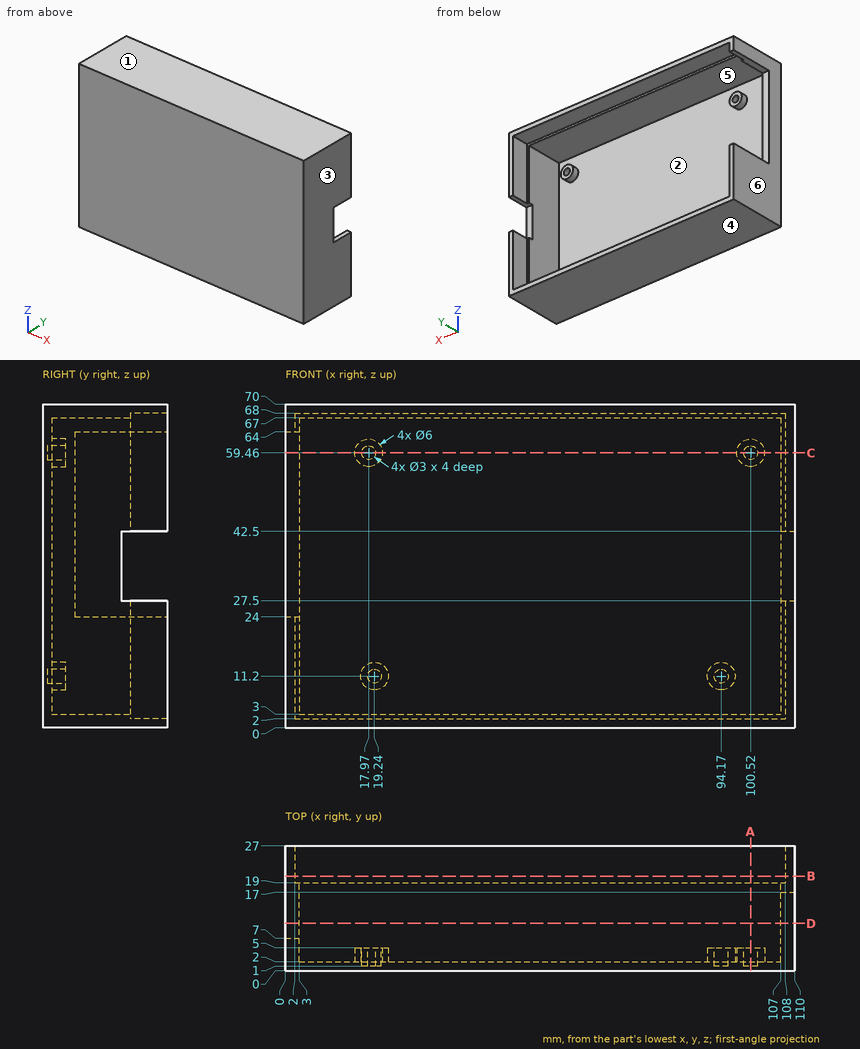
For this review, use the dimensioned drawing (mm, ordinates from the lowest corner) and the shaded views. A direction names the side the tool comes from. Coordinates: 2 decimals unless noted, no trailing zeros. Order: outer loops, then holes, each group sorted by start corner. A loop starts at its lowest first (then second) coordinate and runs counter-clockwise, first axis right, second up. Notation, with made-up numbers: (-9.75, 55.25) - (18.25, 55.25) arc R23 ccw to (18.25, 90.25) - close; hole circle Ø2 at (40.5, -28). An arc over 180 degrees is marked (long way). Use one line per item in the form item = value.
Q1. For probe 1 along X at (y, z) = (2.05, 11.2); probe 2 along X at (y, z) = (2.55, 59.46); probe 3 along X at (y, z) = (1.9, 11.2), list the stretches that pass through material, from the lowest coordinate up. Write a range as from..to.
Checked values:
probe_1 = 0..3, 16.24..17.74, 20.74..22.24, 91.17..92.67, 95.67..97.17, 107..110
probe_2 = 0..3, 14.97..16.47, 19.47..20.97, 97.52..99.02, 102.02..103.52, 107..110
probe_3 = 0..17.74, 20.74..92.67, 95.67..110
Q2. For the marked faces 5 and 6, list the 3-axis set-ups (+Z, -Z, +X, -X, +Y, -Y) from which the entire face can be reached by the end or side of a thin tool; tool diameter is ignored.
Checked values:
face_5 = +Y
face_6 = +Z, -Z, -X, +Y, -Y
Q3. Consider section B-B (y = 20.5). Give the boundary of the cut face in (x, z).
Checked values:
outline = (0, 0) - (110, 0) - (110, 27.5) - (108, 27.5) - (108, 2) - (2, 2) - (2, 24) - (0, 24) - close; (0, 64) - (2, 64) - (2, 68) - (108, 68) - (108, 42.5) - (110, 42.5) - (110, 70) - (0, 70) - close
Q4. Draft analysis for pull direction Z (two halves, no side actions). For the marked faces 1, 2, 3 and 4, state which applies: +Z half, -Z half, draft (parallel to the pull), parting line (faces both ways), or undercut.
Checked values:
face_1 = +Z half
face_2 = undercut
face_3 = draft
face_4 = -Z half
Q5. For P1, Ø1.5, axis at x = 17.5, z = 59, coming from the +Y side; P2, Ø5, axis at x = 70, z = 23.5, coming from the +Y side; P3, Ø3.5, axis at x = 100.5, z = 59, coming from the +Y side, all flat-tipped, find the tip position at first contact; note any pin that passes through.
Checked values:
P1 = 1
P2 = 2
P3 = 5
Q6. Consider section A-A (x = 100.52). Give the boundary of the cut face in (y, z).
Checked values:
outline = (0, 0) - (27, 0) - (27, 2) - (19, 2) - (19, 3) - (2, 3) - (2, 56.46) - (5, 56.46) - (5, 57.96) - (1, 57.96) - (1, 60.96) - (5, 60.96) - (5, 62.46) - (2, 62.46) - (2, 67) - (19, 67) - (19, 68) - (27, 68) - (27, 70) - (0, 70) - close
Q7. Consider section D-D (y = 10.25). Give the boundary of the cut face in (x, z), then the cut area to 3 significant figures.
Checked values:
outline = (0, 0) - (110, 0) - (110, 70) - (0, 70) - (0, 64) - (3, 64) - (3, 67) - (107, 67) - (107, 3) - (3, 3) - (3, 24) - (0, 24) - close
area = 924 mm2
Q8. Consider section C-C (z = 59.46). Give the boundary of the cut face in (x, y), then the cut area to 3 significant figures.
Checked values:
outline = (0, 0) - (110, 0) - (110, 27) - (108, 27) - (108, 19) - (107, 19) - (107, 2) - (103.52, 2) - (103.52, 5) - (102.02, 5) - (102.02, 1) - (99.02, 1) - (99.02, 5) - (97.52, 5) - (97.52, 2) - (20.97, 2) - (20.97, 5) - (19.47, 5) - (19.47, 1) - (16.47, 1) - (16.47, 5) - (14.97, 5) - (14.97, 2) - (3, 2) - (3, 7) - (0, 7) - close
area = 314 mm2
